Build history of the part. All positions in model axes, mm. A direction names the side the tool comes from. Give positions to 0.01 mm unless a question says otherwise; leave off trailing zeros. Order: outer loops, then holes, each group sorted by start corner. A loop starts at its lowest first (then second) coordinate and runs counter-clockwise, first axis right, second up. Notation, with made-up numbers: (-25.75, -39.75) - (6.25, -39.75) arc R4 ccw to (6.25, -35.75) - close; hole circle Ø6 at (64.25, 18.5). An arc over 180 degrees is marked (long way). Write each question's results on one line, items separated by ' | '. Start each with the question number.
1) Cut at A-A on y = -0.25. List the corners of the cut face in (x, z), plus the area to 3 significant figures.
2) Tool access for faces 1 (the face through (3, 2, 1.45)), 2 (the face through (1.45, 2, -3)), 3 (the face through (-1.45, 2, -3)), 4 (the face through (-3, 2, 1.45)), 5 (the face through (1.2, 0, 1.2)): list every direction of +Z, -Z, +X, -X, +Y, -Y with a clear straight run to the whole face (end or side of a thin tool).
3) Drill centre lines: line 1 along Z through (x, y) = (-2, 3); line 2 along Z through (x, y) = (-3.25, 1.5). Where is each one in solid material? Low to high. Write a range as from..to.
4) Drop flat-ended pins along their axis: pin 1 Ø3 at (x, y) = (3.5, 2.5) entering from +Z; pin 2 Ø4 at (x, z) = (-2.5, 1.5) entering from +Y; pin 3 Ø1.5 at (x, y) = (2, 3) entering from -Z. Give the stop position or say it passes through.
from build123d import *

# Parameters (mm, degrees)
SKETCH3_W          = 1.45
SKETCH3_H          = 2
CUT_EXTRUDE1_REACH = 7


with BuildPart() as part:
    # Sketch3 → Revolve1 (revolve)
    with BuildSketch(Plane.XY):
        with BuildLine():
            add(Edge.make_bspline(
                [(5, 0), (3.201562119, 5), (0, 5)],
                knots=[0, 0, 0, 1, 1, 1], degree=2))
            Line((0, 5), (0, 0.5))
            Line((0, 0.5), (0, 0))
            Line((0, 0), (1.45, 0))
            Line((1.45, 0), (2.5, 0))
            Line((2.5, 0), (5, 0))
        make_face()
        with BuildLine():
            add(Edge.make_bspline(
                [(5, 0), (3.201562119, 5), (0, 5)],
                knots=[0, 0, 0, 1, 1, 1], degree=2))
            Line((0, 5), (0, 0.5))
            Line((0, 0.5), (0, 0))
            Line((0, 0), (1.45, 0))
            Line((1.45, 0), (2.5, 0))
            Line((2.5, 0), (5, 0))
        make_face()
        with Locations((0.725, -1)):
            Rectangle(SKETCH3_W, SKETCH3_H)
    revolve(axis=Axis((0, 5, 0), (0, -1, 0)))

    # Sketch5 → Cut-Extrude1 (cut, up to next)
    with BuildSketch(Plane.XZ, mode=Mode.PRIVATE) as cut_extrude1_sk1:
        with BuildLine():
            Line((-2.2, 2.2), (-1.45, 2.2))
            Line((-1.45, 2.2), (-1.45, 4.785133227))
            ThreePointArc((-1.45, 4.785133227), (-3.535533906, 3.535533906), (-4.785133227, 1.45))
            Line((-4.785133227, 1.45), (-2.2, 1.45))
            Line((-2.2, 1.45), (-2.2, 2.2))
        make_face()
    cut_extrude1_tool1 = extrude(cut_extrude1_sk1.sketch, amount=-CUT_EXTRUDE1_REACH, mode=Mode.PRIVATE) & part.part
    add(cut_extrude1_tool1.solids().sort_by_distance((-2.819915, 0, 2.819915))[0], mode=Mode.SUBTRACT)
    # Sketch5 → Cut-Extrude1 (cut, up to next)
    with BuildSketch(Plane.XZ, mode=Mode.PRIVATE) as cut_extrude1_sk2:
        with BuildLine():
            Line((1.45, 2.2), (2.2, 2.2))
            Line((2.2, 2.2), (2.2, 1.45))
            Line((2.2, 1.45), (4.785133227, 1.45))
            ThreePointArc((4.785133227, 1.45), (3.535533906, 3.535533906), (1.45, 4.785133227))
            Line((1.45, 4.785133227), (1.45, 2.2))
        make_face()
    cut_extrude1_tool2 = extrude(cut_extrude1_sk2.sketch, amount=-CUT_EXTRUDE1_REACH, mode=Mode.PRIVATE) & part.part
    add(cut_extrude1_tool2.solids().sort_by_distance((2.819915, 0, 2.819915))[0], mode=Mode.SUBTRACT)
    # Sketch5 → Cut-Extrude1 (cut, up to next)
    with BuildSketch(Plane.XZ, mode=Mode.PRIVATE) as cut_extrude1_sk3:
        with BuildLine():
            Line((4.785133227, -1.45), (2.2, -1.45))
            Line((2.2, -1.45), (2.2, -2.2))
            Line((2.2, -2.2), (1.45, -2.2))
            Line((1.45, -2.2), (1.45, -4.785133227))
            ThreePointArc((1.45, -4.785133227), (3.535533906, -3.535533906), (4.785133227, -1.45))
        make_face()
    cut_extrude1_tool3 = extrude(cut_extrude1_sk3.sketch, amount=-CUT_EXTRUDE1_REACH, mode=Mode.PRIVATE) & part.part
    add(cut_extrude1_tool3.solids().sort_by_distance((2.819915, 0, -2.819915))[0], mode=Mode.SUBTRACT)
    # Sketch5 → Cut-Extrude1 (cut, up to next)
    with BuildSketch(Plane.XZ, mode=Mode.PRIVATE) as cut_extrude1_sk4:
        with BuildLine():
            Line((-2.2, -2.2), (-2.2, -1.45))
            Line((-2.2, -1.45), (-4.785133227, -1.45))
            ThreePointArc((-4.785133227, -1.45), (-3.535533906, -3.535533906), (-1.45, -4.785133227))
            Line((-1.45, -4.785133227), (-1.45, -2.2))
            Line((-1.45, -2.2), (-2.2, -2.2))
        make_face()
    cut_extrude1_tool4 = extrude(cut_extrude1_sk4.sketch, amount=-CUT_EXTRUDE1_REACH, mode=Mode.PRIVATE) & part.part
    add(cut_extrude1_tool4.solids().sort_by_distance((-2.819915, 0, -2.819915))[0], mode=Mode.SUBTRACT)


solid = part.part
Results:
1) outline: circle Ø2.9 at (0, 0) | area: 6.61 mm^2
2) face 1: +Z, +X, +Y, -Y | face 2: -Z, +X, +Y, -Y | face 3: -Z, -X, +Y, -Y | face 4: +Z, -X, +Y, -Y | face 5: -Y
3) line 1: -2.2..2.2 | line 2: -1.45..1.45
4) pin 1: z = 2.2 | pin 2: y = 4.89 | pin 3: z = -3.55
